from build123d import *

# Parameters (mm, degrees)
SKETCH2_W           = 304
SKETCH2_H           = 12
SKETCH2_R           = 10
BOSS_EXTRUDE2_DEPTH = 2
SKETCH4_W           = 2
SKETCH4_H           = 10
SKETCH4_H_2         = 2
BOSS_EXTRUDE4_DEPTH = 2


with BuildPart() as part:
    # Sketch2 → Boss-Extrude2 (new body)
    # profile 1 of 3: a face of its own
    with BuildSketch(Plane(origin=(0, 0, 0), x_dir=(1, 0, 0), z_dir=(0, 1, 0))):
        Rectangle(SKETCH2_W, SKETCH2_H)
    # profile 2 of 3: a face of its own
    with BuildSketch(Plane(origin=(0, 0, 0), x_dir=(1, 0, 0), z_dir=(0, 1, 0))):
        with BuildLine():
            Line((30, -6), (-30, -6))
            ThreePointArc((-30, -6), (-19.831001195, -13.285363729), (-15.97933301, -25.187032248))
            ThreePointArc((-15.97933301, -25.187032248), (0, -10), (15.97933301, -25.187032248))
            ThreePointArc((15.97933301, -25.187032248), (19.831001195, -13.285363729), (30, -6))
        make_face()
    # profile 3 of 3: a face of its own
    with BuildSketch(Plane(origin=(0, 0, 0), x_dir=(1, 0, 0), z_dir=(0, 1, 0))):
        with BuildLine():
            ThreePointArc((15.97933301, -25.187032248), (0, -10), (-15.97933301, -25.187032248))
            ThreePointArc((-15.97933301, -25.187032248), (-15.985534015, -25.593621179), (-16, -26))
            ThreePointArc((-16, -26), (0, -42), (16, -26))
            ThreePointArc((16, -26), (15.985534015, -25.593621179), (15.97933301, -25.187032248))
        make_face()
        with Locations(Location((0, -26, 0), (0, 0, 270))):
            Circle(SKETCH2_R, mode=Mode.SUBTRACT)
    extrude(amount=-BOSS_EXTRUDE2_DEPTH)

    # Sketch4 → Boss-Extrude4 (add)
    with BuildSketch(Plane(origin=(0, 0, 0), x_dir=(1, 0, 0), z_dir=(0, 1, 0))):
        with Locations((-151, 1)):
            Rectangle(SKETCH4_W, SKETCH4_H)
        with Locations((-151, -5)):
            Rectangle(SKETCH4_W, SKETCH4_H_2)
        Polygon((0, -4), (-150, -4), (-150, -6), (-30, -6), (0, -6), align=None)
        Polygon((150, -4), (0, -4), (0, -6), (30, -6), (150, -6), align=None)
        with Locations((151, -5)):
            Rectangle(SKETCH4_W, SKETCH4_H_2)
        with Locations((151, 1)):
            Rectangle(SKETCH4_W, SKETCH4_H)
    extrude(amount=BOSS_EXTRUDE4_DEPTH)


solid = part.part
Can you work these out from the model? Positions are in its coordinate system, mm. Coordinates: 2 decimals unless noted, no trailing zeros. Loops run counter-clockwise (first coordinate to the right, second up) from the corner with the lowest first, then second, coordinate; pieces in that order, holes last. Notation, with made-up numbers: M -8,68 L 37,68 A20 ccw 37,94 Z; hole C 76.25,37 d6. An arc over 180 degrees is marked long. Return JSON: item names as keys, results as strings. Group by question number.
Item 1: Imagine slicing it at B-B (y = -0.8). Please give me the cut outline in (x, z), and give its area (3 significant figures).
Item 2: Imagine slicing it at A-A (x = 0). Please give me the cut outline in (y, z), and give its area (3 significant figures).
Item 3: I'm going to push flat-ended pins straight in: pin 1 Ø1 at (x, z) = (-13.5, 14) entering from +Y; pin 2 Ø1.5 at (x, y) = (83, 0.5) entering from +Z; pin 3 Ø2 at (x, y) = (-2, 0.5) entering from +Z. Where does each tip first touch, or does it pass through?
Item 4: Thinking about a two-plate mould opening in X: for faces 1 (the flat face through (-0.4, 0, 15.7)), 2 (the cylindrical face through (0, -1, 42)), 3 (the flat face through (-2, 0, -1)), which applies, released by +X, released by -X, zero draft, split by the parting line, or undercut?
Item 5: If I drill on L1, parallel to X at y = -0.85, z = 26; L2, parallel to Z at x = -103.5, y = 1.2; L3, parallel to Z at x = -140, y = -1.75, over which ranges is the centre line in solid material (lowest first)? Write a range as from..to.
Item 6: Imagine slicing it at D-D (x = -84). Please give me the cut outline in (y, z), and give its area (3 significant figures).
Item 7: Imagine slicing it at C-C (z = 22.5). Please give me the cut outline in (x, y), and give its area (3 significant figures).
Verdict:
{
 "1": {"outline": "M -152,-6 L 152,-6 L 152,6 L 30,6 A20 cw 16,26 A16 ccw -16,26 A20 cw -30,6 L -152,6 Z; hole C 0,26 d20", "area": "4,520 mm^2"},
 "2": {"outline": "M -2,-6 L 0,-6 L 0,4 L 2,4 L 2,6 L 0,6 L 0,16 L -2,16 Z; M -2,36 L 0,36 L 0,42 L -2,42 Z", "area": "60.0 mm^2"},
 "3": {"pin 1": "stops at y = 0", "pin 2": "stops at z = 6", "pin 3": "stops at z = 41.96"},
 "4": {"face 1": "zero draft", "face 2": "split by the parting line", "face 3": "undercut"},
 "5": {"L1": "x = -16..-10, 10..16", "L2": "z = 4..6", "L3": "z = -6..6"},
 "6": {"outline": "M -2,-6 L 0,-6 L 0,4 L 2,4 L 2,6 L -2,6 Z", "area": "28.0 mm^2"},
 "7": {"outline": "M -16.15,-2 L -9.37,-2 L -9.37,0 L -16.15,0 Z; M 9.37,-2 L 16.15,-2 L 16.15,0 L 9.37,0 Z", "area": "27.1 mm^2"}
}
